The model under review builds one solid part; all positions refer to its coordinate system, in mm. Face numbers are marked on the shaded views. A direction names the side the tool comes from. Coordinates: 2 decimals unless noted, no trailing zeros. Order: outer loops, then holes, each group sorted by start corner. A loop starts at its lowest first (then second) coordinate and runs counter-clockwise, first axis right, second up.
```python
from build123d import *

# Parameters (mm, degrees)
F0_W     = 14
F0_H     = 3
F0_W_2   = 3
F1_DEPTH = 20
F2_DEPTH = 3
F3_W     = 3
F3_H     = 3
F4_DEPTH = 100
F5_W     = 3
F5_H     = 3.5
F6_DEPTH = 100
F7_R     = 1.5
F9_DEPTH = 1


with BuildPart() as f1:
    # F0 (on Front) → F1 (new body)
    with BuildSketch(Plane.XZ):
        Polygon((10, 1.5), (10, 4.5), (-10, 4.5), (-10, 1.5), (-7, 1.5), (7, 1.5), align=None)
        Rectangle(F0_W, F0_H)
        with Locations((11.5, 0)):
            Rectangle(F0_W_2, F0_H)
        with Locations((8.5, 0)):
            Rectangle(F0_W_2, F0_H)
        with Locations((-8.5, 0)):
            Rectangle(F0_W_2, F0_H)
        Polygon((10, -4.5), (10, -1.5), (7, -1.5), (-7, -1.5), (-10, -1.5), (-10, -4.5), align=None)
    extrude(amount=-F1_DEPTH)

    # F0 (on Front) → F2 (join)
    with BuildSketch(Plane.XZ):
        with Locations((-8.5, 0)):
            Rectangle(F0_W_2, F0_H)
        Rectangle(F0_W, F0_H)
        with Locations((8.5, 0)):
            Rectangle(F0_W_2, F0_H)
        with Locations((11.5, 0)):
            Rectangle(F0_W_2, F0_H)
    extrude(amount=F2_DEPTH)

    # F3 (on face) → F4 (cut)
    with BuildSketch(Plane.YZ.offset(13)):
        Polygon((23, -1.75), (23, 1.75), (17, 1.75), (17, 1.5), (20, 1.5), (20, -1.5), (17, -1.5), (17, -1.75), align=None)
        with Locations((18.5, 0)):
            Rectangle(F3_W, F3_H)
    extrude(amount=-F4_DEPTH, mode=Mode.SUBTRACT)

    # F5 (on face) → F6 (cut)
    with BuildSketch(Plane(origin=(0, 17, 0), x_dir=(-1, 0, 0), z_dir=(0, 1, 0))):
        with Locations((11.5, 0)):
            Rectangle(F5_W, F5_H)
        with Locations((8.5, 0)):
            Rectangle(F5_W, F5_H)
    extrude(amount=-F6_DEPTH, mode=Mode.SUBTRACT)

    # F7
    f7_edges = [f1.edges().sort_by_distance(p)[0] for p in [
        (-7, -3, 0),
        (13, -3, 0),
        (10, 0, 3),
        (10, 0, -3),
        (-10, 0, -3.125),
        (-10, 0, 3.125),
        (-7, 17, 0),
        (-10, 20, 3.125),
        (-10, 20, -3.125),
        (13, 17, 0),
        (10, 20, 3.125),
        (10, 20, -3.125),
    ]]
    fillet(f7_edges, radius=F7_R)

    # F8 (on face) → F9 (cut)
    with BuildSketch(Plane.XY.offset(4.5)):
        with BuildLine():
            Line((-2.8206877235, 3), (1.0255347449, 3))
            add(Edge.make_bspline(
                [(2.9492867111, 3.8917100694), (2.1647599693, 3.2639125757), (1.0255347449, 3)],
                knots=[0, 0, 0, 0.5796214889, 0.5796214889, 0.5796214889], degree=2))
            add(Edge.make_bspline(
                [(4.3028023361, 6.85546875), (4.3028023361, 4.9748263889), (2.9492867111, 3.8917100694)],
                knots=[0, 0, 0, 1, 1, 1], degree=2))
            add(Edge.make_bspline(
                [(3.5812311556, 9.1477864583), (4.3028023361, 8.2135416667), (4.3028023361, 6.85546875)],
                knots=[0, 0, 0, 1, 1, 1], degree=2))
            add(Edge.make_bspline(
                [(0.9121773361, 11.0147569444), (2.859659975, 10.08203125), (3.5812311556, 9.1477864583)],
                knots=[0, 0, 0, 1, 1, 1], degree=2))
            add(Edge.make_bspline(
                [(-0.9517549555, 11.9869791667), (-0.558308775, 11.7165798611), (0.9121773361, 11.0147569444)],
                knots=[0, 0, 0, 1, 1, 1], degree=2))
            add(Edge.make_bspline(
                [(-1.5259737055, 12.5475260417), (-1.3452011361, 12.2573784722), (-0.9517549555, 11.9869791667)],
                knots=[0, 0, 0, 1, 1, 1], degree=2))
            add(Edge.make_bspline(
                [(-1.706746275, 13.2265625), (-1.706746275, 12.8376736111), (-1.5259737055, 12.5475260417)],
                knots=[0, 0, 0, 1, 1, 1], degree=2))
            add(Edge.make_bspline(
                [(-1.2601316916, 14.2413194444), (-1.706746275, 13.8524305556), (-1.706746275, 13.2265625)],
                knots=[0, 0, 0, 1, 1, 1], degree=2))
            add(Edge.make_bspline(
                [(0.0219863639, 14.6302083333), (-0.8135171083, 14.6302083333), (-1.2601316916, 14.2413194444)],
                knots=[0, 0, 0, 1, 1, 1], degree=2))
            add(Edge.make_bspline(
                [(1.4499377528, 14.4494357639), (0.7238092806, 14.6302083333), (0.0219863639, 14.6302083333)],
                knots=[0, 0, 0, 1, 1, 1], degree=2))
            add(Edge.make_bspline(
                [(3.2880453917, 13.8129340278), (2.176066225, 14.2686631944), (1.4499377528, 14.4494357639)],
                knots=[0, 0, 0, 1, 1, 1], degree=2))
            Line((3.2880453917, 13.8129340278), (4.2359620584, 16.1037326389))
            add(Edge.make_bspline(
                [(2.1806235167, 16.8237847222), (3.1634794195, 16.5685763889), (4.2359620584, 16.1037326389)],
                knots=[0, 0, 0, 1, 1, 1], degree=2))
            add(Edge.make_bspline(
                [(0.1161703917, 17.0789930556), (1.1977676139, 17.0789930556), (2.1806235167, 16.8237847222)],
                knots=[0, 0, 0, 1, 1, 1], degree=2))
            add(Edge.make_bspline(
                [(-3.3352184972, 16.0262586806), (-2.0865205805, 17.0789930556), (0.1161703917, 17.0789930556)],
                knots=[0, 0, 0, 1, 1, 1], degree=2))
            add(Edge.make_bspline(
                [(-4.5839164139, 13.1293402778), (-4.5839164139, 14.9735243056), (-3.3352184972, 16.0262586806)],
                knots=[0, 0, 0, 1, 1, 1], degree=2))
            add(Edge.make_bspline(
                [(-4.2041421083, 11.421875), (-4.5839164139, 12.1540798611), (-4.5839164139, 13.1293402778)],
                knots=[0, 0, 0, 1, 1, 1], degree=2))
            add(Edge.make_bspline(
                [(-3.1878660666, 10.1397569444), (-3.8243678027, 10.6896701389), (-4.2041421083, 11.421875)],
                knots=[0, 0, 0, 1, 1, 1], degree=2))
            add(Edge.make_bspline(
                [(-1.2813990527, 8.9913194444), (-2.5513643305, 9.58984375), (-3.1878660666, 10.1397569444)],
                knots=[0, 0, 0, 1, 1, 1], degree=2))
            add(Edge.make_bspline(
                [(0.5187311556, 8.0509982639), (0.0766738639, 8.3441840278), (-1.2813990527, 8.9913194444)],
                knots=[0, 0, 0, 1, 1, 1], degree=2))
            add(Edge.make_bspline(
                [(1.1886530306, 7.4388020833), (0.9607884473, 7.7578125), (0.5187311556, 8.0509982639)],
                knots=[0, 0, 0, 1, 1, 1], degree=2))
            add(Edge.make_bspline(
                [(1.4165176139, 6.7126736111), (1.4165176139, 7.1197916667), (1.1886530306, 7.4388020833)],
                knots=[0, 0, 0, 1, 1, 1], degree=2))
            add(Edge.make_bspline(
                [(0.8985054611, 5.611328125), (1.4165176139, 5.98046875), (1.4165176139, 6.7126736111)],
                knots=[0, 0, 0, 1, 1, 1], degree=2))
            add(Edge.make_bspline(
                [(-0.585652525, 5.2421875), (0.3804933084, 5.2421875), (0.8985054611, 5.611328125)],
                knots=[0, 0, 0, 1, 1, 1], degree=2))
            add(Edge.make_bspline(
                [(-2.3675535666, 5.4973958333), (-1.3938122472, 5.2421875), (-0.585652525, 5.2421875)],
                knots=[0, 0, 0, 1, 1, 1], degree=2))
            add(Edge.make_bspline(
                [(-4.7449407194, 6.3815104167), (-3.3412948861, 5.7526041667), (-2.3675535666, 5.4973958333)],
                knots=[0, 0, 0, 1, 1, 1], degree=2))
            Line((-4.7449407194, 6.3815104167), (-4.7449407194, 3.6471354167))
            add(Edge.make_bspline(
                [(-2.8206877235, 3), (-3.8532452246, 3.2092209032), (-4.7449407194, 3.6471354167)],
                knots=[0.477766543, 0.477766543, 0.477766543, 1, 1, 1], degree=2))
        make_face()
    extrude(amount=-F9_DEPTH, mode=Mode.SUBTRACT)


solid = f1.part
```
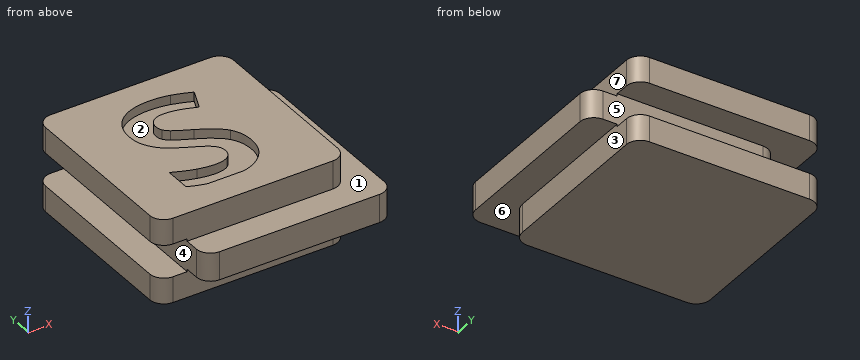
(1) Draft analysis for pull direction X (two halves, no side actions). For the marked faces 1, 2 and 3, state which applies: released by +X, released by -X, zero draft, split by the parting line, or undercut.
A:
face 1: zero draft
face 2: undercut
face 3: released by +X
(2) For pin 1 Ø0.8 at (y, z) = (5.5, 4) entering from +X, flat-tipped, find the tip position at first contact; note if it passes through.
A:
pin 1: stops at x = 10
(3) Wall thickness on probe 1 along Z at (x, y) = (6.5, 18.25); probe 2 along Z at (x, y) = (9.25, -0.75); probe 3 along Y at (x, z) = (4.5, -0.75): over which ranges is each line inside the solid? List them lowest first.
A:
probe 1: z = -4.5 to -1.75, 1.75 to 4.5
probe 2: z = -1.5 to 1.5
probe 3: y = -3 to 17
(4) We need section A-A, the plane x = -8. Write out the cut boundary in (y, z), and give its area (3 significant figures).
A:
outline: (0, -4.5) - (20, -4.5) - (20, -1.75) - (0, -1.75) - close; (0, 1.75) - (20, 1.75) - (20, 4.5) - (0, 4.5) - close
area: 110 mm2
(5) We need section D-D, the plane x = 11. Write out the cut boundary in (y, z), and give its area (3 significant figures).
A:
outline: (-3, -1.5) - (17, -1.5) - (17, 1.5) - (-3, 1.5) - close
area: 60.0 mm2
(6) We need section B-B, the plane z = -3.75. Write out the cut boundary in (x, y).
A:
outline: (-10, 1.5) arc R1.5 ccw to (-8.5, 0) - (8.5, 0) arc R1.5 ccw to (10, 1.5) - (10, 18.5) arc R1.5 ccw to (8.5, 20) - (-8.5, 20) arc R1.5 ccw to (-10, 18.5) - close
(7) Machinability: for the marked faces 4, 5, 6 and 7, which of the approach directions +Z, -Z, +X, -X, +Y, -Y give a long, thin tool a straight path to every point of the face, cutting with its end or side? Answer none if there is none.
A:
face 4: -X, +Y, -Y
face 5: +X, -X, +Y
face 6: -Z, +X, -Y
face 7: +Z, +X, +Y, -Y
(8) We need section C-C, the plane x = 6. Write out the cut boundary in (y, z), and give its area (4 significant figures).
A:
outline: (-3, -1.5) - (0, -1.5) - (0, -4.5) - (20, -4.5) - (20, -1.75) - (17, -1.75) - (17, 1.75) - (20, 1.75) - (20, 4.5) - (0, 4.5) - (0, 1.5) - (-3, 1.5) - close
area: 178.5 mm2
